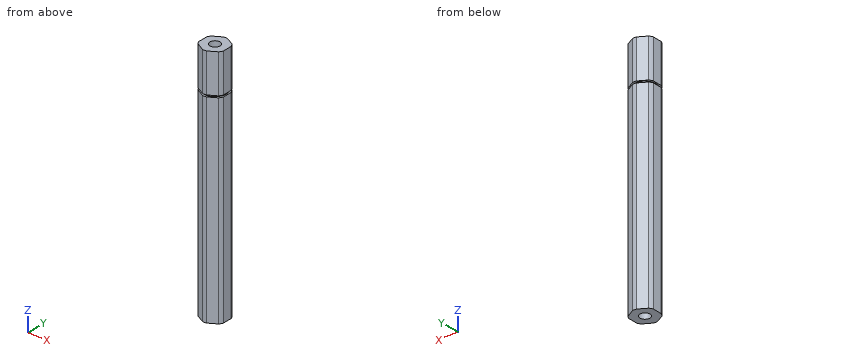
from build123d import *

# Parameters (mm, degrees)
BOSS_EXTRUDE1_DEPTH = 46.76775
SKETCH2_R           = 2.0193
CUT_EXTRUDE1_DEPTH  = 19.05
SKETCH4_R           = 6.35
SKETCH4_R_2         = 4.2926
CUT_EXTRUDE2_DEPTH  = 0.6858


with BuildPart() as part:
    # Sketch1 → Boss-Extrude1 (new, symmetric)
    with BuildSketch(Plane.XY):
        with BuildLine():
            ThreePointArc((4.7625, 1.891713919), (4.43790388, 2.562225), (4.019522311, 3.178589026))
            Line((4.019522311, 3.178589026), (0.742977689, 5.070302945))
            ThreePointArc((0.742977689, 5.070302945), (0, 5.12445), (-0.742977689, 5.070302945))
            Line((-0.742977689, 5.070302945), (-4.019522311, 3.178589026))
            ThreePointArc((-4.019522311, 3.178589026), (-4.43790388, 2.562225), (-4.7625, 1.891713919))
            Line((-4.7625, 1.891713919), (-4.7625, -1.891713919))
            ThreePointArc((-4.7625, -1.891713919), (-4.43790388, -2.562225), (-4.019522311, -3.178589026))
            Line((-4.019522311, -3.178589026), (-0.742977689, -5.070302945))
            ThreePointArc((-0.742977689, -5.070302945), (0, -5.12445), (0.742977689, -5.070302945))
            Line((0.742977689, -5.070302945), (4.019522311, -3.178589026))
            ThreePointArc((4.019522311, -3.178589026), (4.43790388, -2.562225), (4.7625, -1.891713919))
            Line((4.7625, -1.891713919), (4.7625, 1.891713919))
        make_face()
    extrude(amount=BOSS_EXTRUDE1_DEPTH, both=True)

    # Sketch2 → Cut-Extrude1 (cut)
    with BuildSketch(Plane(origin=(0, 0, -46.76775), x_dir=(-1, 0, 0), z_dir=(0, 0, -1))):
        Circle(SKETCH2_R)
    cut_extrude1 = extrude(amount=-CUT_EXTRUDE1_DEPTH, mode=Mode.SUBTRACT)

    # Mirror1: Cut-Extrude1 across plane
    add(cut_extrude1.mirror(Plane.XY), mode=Mode.SUBTRACT)

    # Sketch4 → Cut-Extrude2 (cut)
    with BuildSketch(Plane(origin=(0, 0, 30.95625), x_dir=(-1, 0, 0), z_dir=(0, 0, -1))):
        Circle(SKETCH4_R)
        Circle(SKETCH4_R_2, mode=Mode.SUBTRACT)
    extrude(amount=-CUT_EXTRUDE2_DEPTH, mode=Mode.SUBTRACT)


solid = part.part
Verification items for the finished model (mm, model axes). Coordinates: 2 decimals unless noted, no trailing zeros. Order: outer loops, then holes, each group sorted by start corner. A loop starts at its lowest first (then second) coordinate and runs counter-clockwise, first axis right, second up. Notation, with made-up numbers: M 33,87 L 56,87 A23 ccw 56,125 Z; hole C 77.5,45 d11. An arc over 180 degrees is marked long. One line per item, written item: value. Start each with the question number.
Item 1: Sectioned sample at B-B on z = 39. Record the cut outline in (x, y), then the cut area to 3 significant figures.
Item 2: Sectioned sample at A-A on y = 0. Record the cut outline in (x, z).
Item 3: Sectioned sample at C-C on z = -4.5. Record the cut outline in (x, y), then the cut area to 3 significant figures.
Item 4: Thickness scan on probe 1 along Y at (x, z) = (0, -38.25); probe 2 along Z at (x, y) = (3.25, 3); probe 3 along Y at (x, z) = (0.75, -34.5). Record the ranges inside material, lowest first.
Item 5: Depth check by flat-ended pin: P1, Ø4, axis at y = -4, z = 28, coming from the +X side. Enter the tip coordinate at first touch or a pass-through.
Calculated:
1. outline: M -4.76,-1.89 A5.12 ccw -4.02,-3.18 L -0.74,-5.07 A5.12 ccw 0.74,-5.07 L 4.02,-3.18 A5.12 ccw 4.76,-1.89 L 4.76,1.89 A5.12 ccw 4.02,3.18 L 0.74,5.07 A5.12 ccw -0.74,5.07 L -4.02,3.18 A5.12 ccw -4.76,1.89 Z; hole C 0,0 d4.04
1. area: 64.2 mm^2
2. outline: M -4.76,-46.77 L -2.02,-46.77 L -2.02,-27.72 L 2.02,-27.72 L 2.02,-46.77 L 4.76,-46.77 L 4.76,30.96 L 4.29,30.96 L 4.29,31.64 L 4.76,31.64 L 4.76,46.77 L 2.02,46.77 L 2.02,27.72 L -2.02,27.72 L -2.02,46.77 L -4.76,46.77 L -4.76,31.64 L -4.29,31.64 L -4.29,30.96 L -4.76,30.96 Z
3. outline: M -4.76,-1.89 A5.12 ccw -4.02,-3.18 L -0.74,-5.07 A5.12 ccw 0.74,-5.07 L 4.02,-3.18 A5.12 ccw 4.76,-1.89 L 4.76,1.89 A5.12 ccw 4.02,3.18 L 0.74,5.07 A5.12 ccw -0.74,5.07 L -4.02,3.18 A5.12 ccw -4.76,1.89 Z
3. area: 77.0 mm^2
4. probe 1: -5.12 to -2.02, 2.02 to 5.12
4. probe 2: -46.77 to 30.96, 31.64 to 46.77
4. probe 3: -5.07 to -1.87, 1.87 to 5.07
5. P1: x = 4.72
